```python
from build123d import *

# Parameters (mm, degrees)
HEX_2_DEPTH = 1.1176


with BuildPart() as part:
    # BodySke → BaseBody (revolve)
    with BuildSketch(Plane.XY):
        with BuildLine():
            Line((8.2042, 0), (8.2042, 1.28016))
            Line((8.2042, 1.28016), (7.73176, 1.7526))
            Line((7.73176, 1.7526), (1.8542, 1.7526))
            Line((1.8542, 1.7526), (1.8542, 3.3274))
            Line((1.8542, 3.3274), (1.4732, 3.3274))
            ThreePointArc((1.4732, 3.3274), (0.616396771, 2.601989501), (0, 1.6637))
            Line((0, 1.6637), (0, 0))
            Line((0, 0), (8.2042, 0))
        make_face()
    revolve(axis=Axis((0, 0, 0), (1, 0, 0)))

    # Sketch2 → PreBroach (revolve, cut)
    with BuildSketch(Plane.XY):
        Polygon((0, 0.9906), (1.1176, 0.9906), (1.689523177, 0), (0, 0), align=None)
    revolve(axis=Axis((0, 0, 0), (1, 0, 0)), mode=Mode.SUBTRACT)

    # Sketch3 → Hex 2 (cut)
    with BuildSketch(Plane(origin=(0, 0, 0), x_dir=(0, 0, -1), z_dir=(1, 0, 0))):
        Polygon((-0.9906, -0.571923177), (-0.9906, 0.571923177), (0, 1.143846353), (0.9906, 0.571923177), (0.9906, -0.571923177), (0, -1.143846353), align=None)
    extrude(amount=HEX_2_DEPTH, mode=Mode.SUBTRACT)


solid = part.part
```
For this review, take the finished solid that the model builds, in its own axes (mm). A direction names the side the tool comes from. Round coordinates to 2 decimals unless told otherwise and drop trailing zeros. Write each loop counter-clockwise with the first axis right and the second up, starting at its lowest first coordinate (ties: lowest second). Pieces come first, ordered by that corner, then holes. Notation, with made-up numbers: (24, -32) - (44, -32) arc R26 ccw to (44, -10) - close; hole circle Ø11 at (82.25, 12). An arc over 180 degrees is marked (long way). Put each result on its own line as item: value.
Q1. Mouldability with a two-part tool opening along Y and no side actions: class faces 4 (the face through (0, -1, -1)), 5 (the face through (0.55, -0.86, 0.49)), 6 (the face through (1.66, -0.72, -3.25)) as released by +Y, released by -Y, zero draft, split by the parting line, or undercut.
Solved:
face 4: zero draft
face 5: undercut
face 6: split by the parting line
Q2. Machinability: for faces 1 (the face through (0.551, -0.854, -0.502)), 2 (the face through (1.854, -1.4, -1.4)), 3 (the face through (8.204, 0, 0)), which of the approach directions +Z, -Z, +X, -X, +Y, -Y give a long, thin tool a straight path to every point of the face, cutting with its end or side? Answer none if there is none.
Solved:
face 1: -X
face 2: +X
face 3: +Z, -Z, +X, +Y, -Y
Q3. Wall thickness on probe 1 along Y at (x, z) = (1, -0.5); probe 2 along Y at (x, z) = (1.5, -1); probe 3 along Z at (x, y) = (6.75, -1.25): over which ranges is each line inside the solid? List them lowest first.
Solved:
probe 1: y = -2.94 to -0.86, 0.86 to 2.94
probe 2: y = -3.17 to 3.17
probe 3: z = -1.23 to 1.23
Q4. We need section B-B (x = 3.75). Give the boundary of the cut face in (y, z), and give its area (3 significant figures).
Solved:
outline: circle Ø3.51 at (0, 0)
area: 9.65 mm2
Q5. Insertion check: pin 1 Ø3 at (x, z) = (5.5, 2.5) entering from -Y; pin 2 Ø1.5 at (y, z) = (-2, 1.5) entering from -X; pin 3 Ø0.6 at (x, y) = (0.5, 0.5) entering from -Z (3 decimals). Each pin has a flat end and moves straight along its axis. Give the tip position at first contact, or say it passes through.
Solved:
pin 1: stops at y = -1.44
pin 2: stops at x = 0.04
pin 3: stops at z = -2.755
Q6. We need section A-A (x = 1). Give the boundary of the cut face in (y, z), and give its area (3 significant figures).
Solved:
outline: circle Ø5.96 at (0, 0); hole (-1.14, 0) - (-0.57, -0.99) - (0.57, -0.99) - (1.14, 0) - (0.57, 0.99) - (-0.57, 0.99) - close
area: 24.5 mm2
Q7. We need section C-C (y = 2.5). Give the boundary of the cut face in (x, z), and give its area (3 significant figures).
Solved:
outline: (1.47, -2.2) - (1.85, -2.2) - (1.85, 2.2) - (1.47, 2.2) arc R3.03 ccw to start
area: 4.54 mm2
Q8. We need section D-D (z = -2). Give the boundary of the cut face in (x, y).
Solved:
outline: (1.47, -2.66) - (1.85, -2.66) - (1.85, 2.66) - (1.47, 2.66) arc R3.38 ccw to start
